Source: CAD feature listing. Evaluate the final solid. Frame: model axes, mm. Face numbers are marked on the shaded views. A direction names the side the tool comes from. Give positions to 0.01 mm unless a question says otherwise; leave off trailing zeros. Loops run counter-clockwise (first coordinate to the right, second up) from the corner with the lowest first, then second, coordinate; pieces in that order, holes last. Notation, with made-up numbers: M -37,-24.75 L -11,-24.75 A4 ccw -11,-20.75 Z; hole C 29,79 d5. An arc over 180 degrees is marked long. Answer in a Markdown table with one row per item.
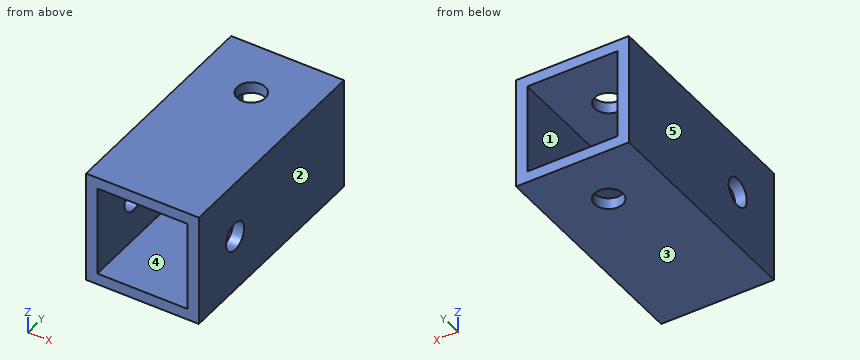
Autodesk Inventor part; units mm, degrees
ref_plane "YZ Plane" through (0, 0, 0) normal (1, 0, 0) x (0, 1, 0)
ref_plane "XZ Plane" through (0, 0, 0) normal (0, 1, 0) x (-1, 0, 0)
ref_plane "XY Plane" through (0, 0, 0) normal (0, 0, 1) x (1, 0, 0)
sketch "スケッチ1" plane through (0, 0, 0) normal (0, 1, 0) x (-1, 0, 0)
  line L0 (0, 0) -> (12, 0)
  line L1 (12, 0) -> (12, -12)
  line L2 (12, -12) -> (0, -12)
  line L3 (0, -12) -> (0, 0)
  line L4 (1.2, -1.2) -> (10.8, -1.2)
  line L5 (10.8, -1.2) -> (10.8, -10.8)
  line L6 (10.8, -10.8) -> (1.2, -10.8)
  line L7 (1.2, -10.8) -> (1.2, -1.2)
  dimension "d0" = 12
  dimension "d1" = 12
  dimension "d2" = 9.6
  dimension "d3" = 9.6
  dimension "d4" = 1.2
  dimension "d5" = 1.2
extrude "押し出し1" add sketch "スケッチ1" along normal blind 24
sketch "スケッチ2" plane through (-12, 0, -12) normal (-1, 0, 0) x (0, 0, 1)
  line L0 (0, 0) -> (12, 0)
  line L1 (0, 0) -> (0, 24)
  point P0 (6, 6)
  dimension "d8" = 6
  dimension "d9" = 6
hole "穴1" at (-12, 6, -6) direction (1, 0, 0) diameter 3 end through all
sketch "スケッチ3" plane through (0, 0, -12) normal (0, 0, -1) x (-1, 0, 0)
  line L0 (0, 0) -> (0, 24)
  line L1 (0, 24) -> (12, 24)
  point P0 (6, 18)
  dimension "d17" = 6
  dimension "d18" = 6
hole "穴2" at (-6, 18, -12) direction (0, 0, 1) diameter 3 end through all
properties part number "前後直動12x12x24" material "アルミニウム 6061"
Q1. Ray query, probe 1 along X at (y, z) = (18, -0.35); probe 2 along Y at (x, z) = (-6, -0.3); probe 3 along Z at (x, y) = (-6.25, 14). Return the intervals inside material, ascending. Write a range as from..to.
Values follow:
| item | result |
|---|---|
| probe 1 | -12..-7.5, -4.5..0 |
| probe 2 | 0..16.5, 19.5..24 |
| probe 3 | -12..-10.8, -1.2..0 |
Q2. Section query C-C (x = -6). Output: boundary loops of the cut face in (y, z).
Values follow:
| item | result |
|---|---|
| outline | M 0,-12 L 16.5,-12 L 16.5,-10.8 L 0,-10.8 Z; M 0,-1.2 L 16.5,-1.2 L 16.5,0 L 0,0 Z; M 19.5,-12 L 24,-12 L 24,-10.8 L 19.5,-10.8 Z; M 19.5,-1.2 L 24,-1.2 L 24,0 L 19.5,0 Z |
Q3. Section query B-B (z = -6). Output: boundary loops of the cut face in (x, y).
Values follow:
| item | result |
|---|---|
| outline | M -12,0 L -10.8,0 L -10.8,4.5 L -12,4.5 Z; M -12,7.5 L -10.8,7.5 L -10.8,24 L -12,24 Z; M -1.2,0 L 0,0 L 0,4.5 L -1.2,4.5 Z; M -1.2,7.5 L 0,7.5 L 0,24 L -1.2,24 Z |
Q4. Section query D-D (x = -3). Output: boundary loops of the cut face in (y, z).
Values follow:
| item | result |
|---|---|
| outline | M 0,-12 L 24,-12 L 24,-10.8 L 0,-10.8 Z; M 0,-1.2 L 24,-1.2 L 24,0 L 0,0 Z |
Q5. Mould query, pull axis Z, two halves, no side actions, for the marked faces 1, 2 and 3. Classes: +Z half, -Z half, draft (parallel to the pull), parting line (faces both ways), or undercut.
Values follow:
| item | result |
|---|---|
| face 1 | undercut |
| face 2 | draft |
| face 3 | -Z half |
Q6. Reachability of the marked faces 4 and 5 from +Z, -Z, +X, -X, +Y, -Y: full face, straight path, thin tool, end or side. Return the list, or none.
Values follow:
| item | result |
|---|---|
| face 4 | +Y, -Y |
| face 5 | +Z, -Z, -X, +Y, -Y |
Q7. Section query A-A (y = 6). Output: boundary loops of the cut face in (x, z).
Values follow:
| item | result |
|---|---|
| outline | M -12,-12 L 0,-12 L 0,-7.5 L -1.2,-7.5 L -1.2,-10.8 L -10.8,-10.8 L -10.8,-7.5 L -12,-7.5 Z; M -12,-4.5 L -10.8,-4.5 L -10.8,-1.2 L -1.2,-1.2 L -1.2,-4.5 L 0,-4.5 L 0,0 L -12,0 Z |
Q8. Contact query for flat-ended pins moving along their axis: pin 1 Ø4 at (x, y) = (-6, 18) entering from +Z; pin 2 Ø2.5 at (y, z) = (6, -6) entering from +X. Output: stop coordinate, or through.
Values follow:
| item | result |
|---|---|
| pin 1 | z = 0 |
| pin 2 | through |
